Can you work these out from the model? Positions are in its coordinate system, mm. Round coordinates to 2 decimals unless told otherwise and drop trailing zeros. Loops run counter-clockwise (first coordinate to the right, second up) from the corner with the lowest first, then second, coordinate; pieces in that order, holes last. Notation, with made-up numbers: M 66.5,53.5 L 94.5,53.5 A15 cw 94.5,76.5 Z; hole C 88.5,62.25 d7. An arc over 180 degrees is marked long. Return JSON: item names as keys, results as strings.
```python
from build123d import *

# Parameters (mm, degrees)
F0_W      = 304.8
F0_H      = 203.2
F1_DEPTH  = 1.5875
F3_DEPTH  = 50.8
F5_DEPTH  = 50.8
F7_DEPTH  = 50.8
F9_DEPTH  = 50.8
F10_DEPTH = 50.8
F12_DEPTH = 50.8
F13_DEPTH = 50.8


with BuildPart() as f1:
    # F0 (on Front) → F1 (new body)
    with BuildSketch(Plane.XZ):
        with Locations((50.476827, 0.969891)):
            Rectangle(F0_W, F0_H)
    extrude(amount=F1_DEPTH)

    # F2 (on face) → F3 (cut)
    with BuildSketch(Plane.XZ.offset(1.5875)):
        with BuildLine():
            Line((15.86265, 62.592995), (14.575709, 53.066764))
            ThreePointArc((14.575709, 53.066764), (50.476827, 17.165645), (86.377946, 53.066764))
            Line((86.377946, 53.066764), (84.91056, 63.225917))
            ThreePointArc((84.91056, 63.225917), (50.147756, 88.966374), (15.86265, 62.592995))
        make_face()
        with BuildLine():
            Line((21.263311, 102.569891), (15.86265, 62.592995))
            ThreePointArc((15.86265, 62.592995), (50.147756, 88.966374), (84.91056, 63.225917))
            Line((84.91056, 63.225917), (79.227723, 102.569891))
            Line((79.227723, 102.569891), (21.263311, 102.569891))
        make_face()
    extrude(amount=-F3_DEPTH, mode=Mode.SUBTRACT)

    # F4 (on face) → F5 (cut)
    with BuildSketch(Plane.XZ.offset(1.5875)):
        with BuildLine():
            ThreePointArc((10.542255, 102.569891), (17.11496, 98.736978), (19.782878, 91.611398))
            Line((19.782878, 91.611398), (21.263311, 102.569891))
            Line((21.263311, 102.569891), (10.542255, 102.569891))
        make_face()
    extrude(amount=-F5_DEPTH, mode=Mode.SUBTRACT)

    # F6 (on face) → F7 (cut)
    with BuildSketch(Plane.XZ.offset(1.5875)):
        with BuildLine():
            ThreePointArc((80.943088, 90.693909), (83.775623, 98.891014), (91.629388, 102.569891))
            Line((91.629388, 102.569891), (79.227723, 102.569891))
            Line((79.227723, 102.569891), (80.943088, 90.693909))
        make_face()
    extrude(amount=-F7_DEPTH, mode=Mode.SUBTRACT)

    # F8 (on face) → F9 (cut)
    with BuildSketch(Plane.XZ.offset(1.5875)):
        with BuildLine():
            Line((-33.738296, 18.680416), (-45.690459, 102.569891))
            Line((-45.690459, 102.569891), (-101.923173, 102.569891))
            Line((-101.923173, 102.569891), (-101.923173, 0))
            ThreePointArc((-101.923173, 0), (-93.593919, 20.108597), (-73.485322, 28.43785))
            ThreePointArc((-73.485322, 28.43785), (-66.705464, 27.617836), (-60.316604, 25.205083))
            Line((-60.316604, 25.205083), (-33.738296, 18.680416))
        make_face()
    extrude(amount=-F9_DEPTH, mode=Mode.SUBTRACT)

    # F8 (on face) → F10 (cut)
    with BuildSketch(Plane.XZ.offset(1.5875)):
        with BuildLine():
            Line((-33.738296, -100.630109), (-33.738296, -23.826821))
            Line((-33.738296, -23.826821), (-66.974824, -27.682571))
            ThreePointArc((-66.974824, -27.682571), (-70.208242, -28.2484), (-73.485322, -28.43785))
            ThreePointArc((-73.485322, -28.43785), (-93.593919, -20.108597), (-101.923173, 0))
            Line((-101.923173, 0), (-101.923173, -100.630109))
            Line((-101.923173, -100.630109), (-33.738296, -100.630109))
        make_face()
    extrude(amount=-F10_DEPTH, mode=Mode.SUBTRACT)

    # F11 (on face) → F12 (cut)
    with BuildSketch(Plane.XZ.offset(1.5875)):
        with BuildLine():
            Line((202.876827, 102.569891), (147.253108, 102.569891))
            Line((147.253108, 102.569891), (140.32495, 17.84187))
            Line((140.32495, 17.84187), (171.340779, 22.817166))
            ThreePointArc((171.340779, 22.817166), (175.049557, 23.719205), (178.854391, 24.022436))
            ThreePointArc((178.854391, 24.022436), (195.840819, 16.986428), (202.876827, 0))
            Line((202.876827, 0), (202.876827, 102.569891))
        make_face()
    extrude(amount=-F12_DEPTH, mode=Mode.SUBTRACT)

    # F11 (on face) → F13 (cut)
    with BuildSketch(Plane.XZ.offset(1.5875)):
        with BuildLine():
            Line((171.950437, -23.008974), (140.32495, -18.366525))
            Line((140.32495, -18.366525), (140.32495, -100.630109))
            Line((140.32495, -100.630109), (202.876827, -100.630109))
            Line((202.876827, -100.630109), (202.876827, 0))
            ThreePointArc((202.876827, 0), (195.840819, -16.986428), (178.854391, -24.022436))
            ThreePointArc((178.854391, -24.022436), (175.365419, -23.76772), (171.950437, -23.008974))
        make_face()
    extrude(amount=-F13_DEPTH, mode=Mode.SUBTRACT)


solid = f1.part
```
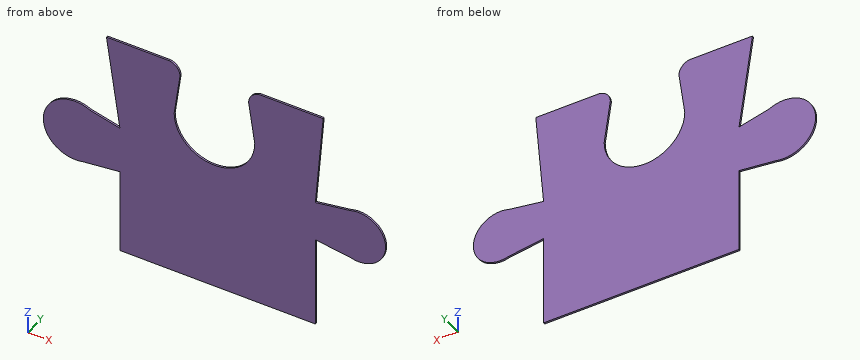
Q1. I'm going to push a flat-ended pin straight in: pin 1 Ø0.8 at (y, z) = (-0.5, -68.5) entering from +X. Where does the tip first touch, or does it pass through?
Results:
{"pin 1": "stops at x = 140.32"}
Q2. Suppose I cut it at D-D, the plane z = -82.5. Please give me the cut outline in (x, y).
Results:
{"outline": "M -33.74,-1.59 L 140.32,-1.59 L 140.32,0 L -33.74,0 Z"}
Q3. Suppose I cut it at B-B, the plane y = -0.8. Please give me the cut outline in (x, z), plus the area to 3 significant figures.
Results:
{"outline": "M -73.49,-28.44 A28.44 ccw -66.97,-27.68 L -33.74,-23.83 L -33.74,-100.63 L 140.32,-100.63 L 140.32,-18.37 L 171.95,-23.01 A24.02 ccw 178.85,-24.02 A24.02 ccw 202.88,0 A24.02 ccw 178.85,24.02 A24.02 ccw 171.34,22.82 L 140.32,17.84 L 147.25,102.57 L 91.63,102.57 A11.14 ccw 80.94,90.69 L 86.38,53.07 A35.9 cw 14.58,53.07 L 19.78,91.61 A11.33 ccw 10.54,102.57 L -45.69,102.57 L -33.74,18.68 L -60.32,25.21 A28.44 ccw -73.49,28.44 A28.44 ccw Z", "area": "36,600 mm2"}
Q4. Suppose I cut it at C-C, the plane x = 59. Please give me the cut outline in (y, z), plus the area to 3 significant figures.
Results:
{"outline": "M -1.59,-100.63 L 0,-100.63 L 0,18.19 L -1.59,18.19 Z", "area": "189 mm2"}
Q5. Suppose I cut it at A-A, the plane z = 37. Please give me the cut outline in (x, y).
Results:
{"outline": "M -36.35,-1.59 L 18.37,-1.59 L 18.37,0 L -36.35,0 Z; M 82.58,-1.59 L 141.89,-1.59 L 141.89,0 L 82.58,0 Z"}
Q6. If I drill on line 1 along X through (y, z) = (-0.95, 94); line 2 along X through (y, z) = (-0.25, 59.5); line 3 along X through (y, z) = (-0.9, -78.5), over which ranges is the centre line in solid material (lowest first)?
Results:
{"line 1": "x = -44.47 to 19.49, 81.22 to 146.55", "line 2": "x = -39.55 to 15.44, 85.45 to 143.73", "line 3": "x = -33.74 to 140.32"}
